from build123d import *

# Parameters (mm, degrees)
SKETCH005_R      = 5.25
EXTRUDE005_DEPTH = 7
SKETCH004_R      = 3.5
EXTRUDE004_DEPTH = 50
EXTRUDE003_DEPTH = 15
FILLET_1_R       = 2
FILLET_2_R       = 1


with BuildPart() as extrude005:
    # Sketch005 (on Face10 of Cut002) → Extrude005 (new body)
    with BuildSketch(Plane.XZ.offset(-14.220068)):
        with Locations((-22.5, 7.5)):
            Circle(SKETCH005_R)
        with Locations((22.5, 7.5)):
            Circle(SKETCH005_R)
    extrude(amount=-EXTRUDE005_DEPTH)


with BuildPart() as extrude004:
    # Sketch004 (on Face5 of Extrude003) → Extrude004 (new body)
    with BuildSketch(Plane.XZ.offset(-14.220068)):
        with Locations((-73, 7.5)):
            Circle(SKETCH004_R)
        with Locations((73, 7.5)):
            Circle(SKETCH004_R)
        with Locations((-22.5, 7.5)):
            Circle(SKETCH004_R)
        with Locations((22.5, 7.5)):
            Circle(SKETCH004_R)
    extrude(amount=-EXTRUDE004_DEPTH)


with BuildPart() as fillet_body:
    # Sketch003 → Extrude003 (new body)
    with BuildSketch(Plane.XY):
        with BuildLine():
            Line((-80, 26.220068), (-25.514702, 26.220068))
            ThreePointArc((-25.514702, 26.220068), (0, 19.220068), (25.514702, 26.220068))
            Line((25.514702, 26.220068), (80, 26.220068))
            Line((80, 26.220068), (80, 14.220068))
            Line((80, 14.220068), (-80, 14.220068))
            Line((-80, 14.220068), (-80, 26.220068))
        make_face()
    extrude(amount=EXTRUDE003_DEPTH)

    # Cut002: cut Extrude004
    add(extrude004.part, mode=Mode.SUBTRACT)

    # Cut003: cut Extrude005
    add(extrude005.part, mode=Mode.SUBTRACT)

    # Fillet 1
    fillet_1_edges = [fillet_body.edges().sort_by_distance(p)[0] for p in [
        (-80, 26.220068, 7.5),
    ]]
    fillet(fillet_1_edges, radius=FILLET_1_R)

    # Fillet 2
    fillet_2_edges = [fillet_body.edges().sort_by_distance(p)[0] for p in [
        (-80, 14.220068, 7.5),
        (80, 26.220068, 7.5),
        (80, 14.220068, 7.5),
    ]]
    fillet(fillet_2_edges, radius=FILLET_2_R)


solid = fillet_body.part
Work out the finished part from the listing and answer in its coordinate system (mm). A direction names the side the tool comes from. Coordinates: 2 decimals unless noted, no trailing zeros. Write each loop counter-clockwise with the first axis right and the second up, starting at its lowest first coordinate (ties: lowest second). Pieces come first, ordered by that corner, then holes. Notation, with made-up numbers: M -33,73.25 L -20,73.25 A23 cw -20,89.25 Z; hole C -8,-5.5 d11. An arc over 180 degrees is marked long. Write item = value, one per line.
1. The part is cut by section A-A (x = -73). Determine the outline of the cut face in (y, z).
Solution:
outline = M 14.22,0 L 26.22,0 L 26.22,4 L 14.22,4 Z; M 14.22,11 L 26.22,11 L 26.22,15 L 14.22,15 Z
2. The part is cut by section D-D (x = 22). Determine the outline of the cut face in (y, z).
Solution:
outline = M 14.22,0 L 24.32,0 L 24.32,4.04 L 21.22,4.04 L 21.22,2.27 L 14.22,2.27 Z; M 14.22,12.73 L 21.22,12.73 L 21.22,10.96 L 24.32,10.96 L 24.32,15 L 14.22,15 Z
3. Flat-ended cylindrical pins translate along their axes: pin 1 (6.5 mm diameter, centred on x = 22.5, z = 7.5, fed in from -Y); pin 2 (1.5 mm diameter, centred on x = -7, z = 8, fed in from +Y); pin 3 (5 mm diameter, centred on x = -22.5, z = 10, fed in from -Y). Find the tip coordinate at first contact, or state that the pin passes through.
Solution:
pin_1 = through
pin_2 = 19.82
pin_3 = 21.22
4. For faces 5 (the face through (1, 19, 0)), 6 (the face through (-21, 21.22, 4)), determine the directions among +Z, -Z, +X, -X, +Y, -Y from which every point of the face is accessible in a straight line to the end or side of a thin tool.
Solution:
face_5 = -Z, +X, -X, +Y, -Y
face_6 = -Y
5. Straight lines are drawn through the part: line 1 (Z direction, x = -73, y = 22.75); line 2 (X direction, y = 23.5, z = 5.5); line 3 (X direction, y = 19, z = 12). For each, find the intervals that lie inside material, in ascending order. Write a range as from..to.
Solution:
line_1 = 0..4, 11..15
line_2 = -80..-75.87, -70.13..-25.37, 25.37..70.13, 75.87..80
line_3 = -80..-25.2, -19.8..19.8, 25.2..80
6. The part is cut by section C-C (x = -22.5). Determine the outline of the cut face in (y, z), then the cut area to 3 significant figures.
Solution:
outline = M 14.22,0 L 24.57,0 L 24.57,4 L 21.22,4 L 21.22,2.25 L 14.22,2.25 Z; M 14.22,12.75 L 21.22,12.75 L 21.22,11 L 24.57,11 L 24.57,15 L 14.22,15 Z
area = 58.3 mm2
7. Determine the mould class of faces 1 (the face through (25.84, 23.13, 8.55)), 2 (the face through (-25.997, 23.13, 7.654)), 3 (the face through (1, 19, 15)), 4 (the face through (80, 20, 7)) for opening direction X: released by +X, released by -X, zero draft, split by the parting line, or undercut.
Solution:
face_1 = undercut
face_2 = undercut
face_3 = zero draft
face_4 = released by +X
8. The part is cut by section B-B (z = 7.5). State how many separate pieces and enclosed holes the cut face has, then the cut area to 3 significant figures.
Solution:
separate_pieces = 5
enclosed_holes = 0
area = 1,310 mm2
